The model under review builds one solid part; all positions refer to its coordinate system, in mm. A direction names the side the tool comes from. Give positions to 0.01 mm unless a question says otherwise; leave off trailing zeros. Order: outer loops, then holes, each group sorted by start corner. A loop starts at its lowest first (then second) coordinate and runs counter-clockwise, first axis right, second up. Notation, with made-up numbers: (3, -31) - (16, -31) arc R26 ccw to (16, -13) - close; hole circle Ø4 at (75, 35). An arc over 180 degrees is marked (long way). Use CSV: the item, a comma, the result in double quotes. Start each with the question number.
1. Take a section at C-C, the plane y = 5.75. Count the separate pieces of the cut face and the enclosed holes in it, then the cut area to 3 significant figures.
2. Machinability: for faces 1 (the cylindrical face through (-0.705, 5.324, 45.673)), 2 (the flat face through (19, 4.4, 53)), 3 (the cylindrical face through (20.755, 5.718, -53.044)), which of the approach directions +Z, -Z, +X, -X, +Y, -Y give a long, thin tool a straight path to every point of the face, cutting with its end or side? Answer none if there is none.
3. Take a section at A-A, the plane x = 0. State the section outline as (y, z) points.
4. For pin 1 (2.5 mm diameter, centred on x = 22.5, z = -49.5, fed in from -Y); pin 2 (2 mm diameter, centred on x = -29, z = -29.5, fed in from +Y); pin 3 (5 mm diameter, centred on x = -1.5, z = 42, fed in from +Y); pin 4 (1.5 mm diameter, centred on y = 3, z = -45.5, fed in from +X), all flat-tipped, find the tip position at first contact; note any pin that passes through.
5. Take a section at B-B, the plane x = 42.5. State the section outline as (y, z) points, then the cut area to 3 significant figures.
6. Take a section at D-D, the plane z = -42.5. State the section outline as (x, y) points, then the cut area to 3 significant figures.
7. Draft analysis for pull direction X (two halves, no side actions). For faces 4 (the flat face through (-28, 0, 28)), 5 (the cylindrical face through (-20.18, 2.17, -46.91)), state which applies: released by +X, released by -X, zero draft, split by the parting line, or undercut.
8. To check wall thickness, follow line 1 (X direction, y = 6.75, z = -19); line 2 (Z direction, x = -52.5, y = 1.75); line 3 (Z direction, x = -31, y = 3.5). State the ranges of each line that lie inside material, in increasing order. Write a range as [from, to].
```python
from build123d import *

# Parameters (mm, degrees)
SKETCH1_R                                           = 65
SKETCH1_R_2                                         = 37.5
BOSS_EXTRUDE1_DEPTH                                 = 7
CBORE_FOR_M3_HEX_SOCKET_HEAD_CAP_SCREW1_D           = 3.4
CBORE_FOR_M3_HEX_SOCKET_HEAD_CAP_SCREW1_CBORE_D     = 6.5
CBORE_FOR_M3_HEX_SOCKET_HEAD_CAP_SCREW1_CBORE_DEPTH = 3.4
CBORE_FOR_M4_HEX_SOCKET_HEAD_CAP_SCREW1_D           = 4.5
CBORE_FOR_M4_HEX_SOCKET_HEAD_CAP_SCREW1_CBORE_D     = 8
CBORE_FOR_M4_HEX_SOCKET_HEAD_CAP_SCREW1_CBORE_DEPTH = 4.4


with BuildPart() as part:
    # Sketch1 → Boss-Extrude1 (new body)
    with BuildSketch(Plane(origin=(0, 0, 0), x_dir=(1, 0, 0), z_dir=(0, 1, 0))):
        with Locations(Location((0, 0, 0), (0, 0, 270))):
            Circle(SKETCH1_R)
        with Locations(Location((0, 0, 0), (0, 0, 270))):
            Circle(SKETCH1_R_2, mode=Mode.SUBTRACT)
    extrude(amount=BOSS_EXTRUDE1_DEPTH)

    # CBORE for M3 Hex Socket Head Cap Screw1 (through all)
    with Locations(Plane(origin=(0, 7, 0), x_dir=(1, 0, 0), z_dir=(0, 1, 0))):
        with Locations((-30.0520382, 30.0520382), (0, 42.5), (30.0520382, 30.0520382), (42.5, 0), (30.0520382, -30.0520382), (0, -42.5), (-30.0520382, -30.0520382), (-42.5, 0)):
            CounterBoreHole(CBORE_FOR_M3_HEX_SOCKET_HEAD_CAP_SCREW1_D / 2, CBORE_FOR_M3_HEX_SOCKET_HEAD_CAP_SCREW1_CBORE_D / 2, CBORE_FOR_M3_HEX_SOCKET_HEAD_CAP_SCREW1_CBORE_DEPTH)

    # CBORE for M4 Hex Socket Head Cap Screw1 (through all)
    with Locations(Plane(origin=(0, 0, 0), x_dir=(-1, 0, 0), z_dir=(0, -1, 0))):
        with Locations((-50.813374288, -21.04758878), (-50.813374288, 21.04758878), (-21.04758878, 50.813374288), (21.04758878, 50.813374288), (50.813374288, 21.04758878), (50.813374288, -21.04758878), (21.04758878, -50.813374288), (-21.04758878, -50.813374288)):
            CounterBoreHole(CBORE_FOR_M4_HEX_SOCKET_HEAD_CAP_SCREW1_D / 2, CBORE_FOR_M4_HEX_SOCKET_HEAD_CAP_SCREW1_CBORE_D / 2, CBORE_FOR_M4_HEX_SOCKET_HEAD_CAP_SCREW1_CBORE_DEPTH)


solid = part.part
```
Determined:
1,separate pieces,"1"
1,enclosed holes,"17"
1,area,"8,460 mm²"
2,face 1,"+Y"
2,face 2,"-Y"
2,face 3,"+Y, -Y"
3,outline,"(0, -65) - (7, -65) - (7, -45.75) - (3.6, -45.75) - (3.6, -44.2) - (0, -44.2) - close; (0, -40.8) - (3.6, -40.8) - (3.6, -39.25) - (7, -39.25) - (7, -37.5) - (0, -37.5) - close; (0, 37.5) - (7, 37.5) - (7, 39.25) - (3.6, 39.25) - (3.6, 40.8) - (0, 40.8) - close; (0, 44.2) - (3.6, 44.2) - (3.6, 45.75) - (7, 45.75) - (7, 65) - (0, 65) - close"
4,pin 1,"stops at y = 4.4"
4,pin 2,"stops at y = 3.6"
4,pin 3,"stops at y = 7"
4,pin 4,"stops at x = 47.14"
5,outline,"(0, -49.18) - (7, -49.18) - (7, -3.25) - (3.6, -3.25) - (3.6, -1.7) - (0, -1.7) - close; (0, 1.7) - (3.6, 1.7) - (3.6, 3.25) - (7, 3.25) - (7, 49.18) - (0, 49.18) - close"
5,area,"654 mm²"
6,outline,"(-49.18, 0) - (-1.7, 0) - (-1.7, 3.6) - (-3.25, 3.6) - (-3.25, 7) - (-49.18, 7) - close; (1.7, 0) - (49.18, 0) - (49.18, 7) - (3.25, 7) - (3.25, 3.6) - (1.7, 3.6) - close"
6,area,"654 mm²"
7,face 4,"zero draft"
7,face 5,"undercut"
8,line 1,"x = [-62.16, -51.75], [-49.88, -32.33], [32.33, 49.88], [51.75, 62.16]"
8,line 2,"z = [-38.32, -24.67], [-17.42, 17.42], [24.67, 38.32]"
8,line 3,"z = [-57.13, -31.46], [-28.64, -21.1], [21.1, 28.64], [31.46, 57.13]"
